```python
from build123d import *


with BuildPart() as part:
    # Эскиз2 → Повернуть1 (revolve)
    with BuildSketch(Plane.XY):
        with BuildLine():
            Line((0, 21), (0, 15))
            ThreePointArc((0, 15), (0.585786438, 13.585786438), (2, 13))
            Line((2, 13), (5, 13))
            Line((5, 13), (5, 14))
            Line((5, 14), (3, 14))
            ThreePointArc((3, 14), (1.585786438, 14.585786438), (1, 16))
            Line((1, 16), (1, 21))
            Line((1, 21), (0, 21))
        make_face()
    revolve(axis=Axis((0, 0, 0), (1, 0, 0)))


solid = part.part
```
Design review of the part built by this model. Coordinates are the model's own, in mm. A direction names the side the tool comes from. Give positions to 0.01 mm unless a question says otherwise; leave off trailing zeros. Order: outer loops, then holes, each group sorted by start corner. A loop starts at its lowest first (then second) coordinate and runs counter-clockwise, first axis right, second up. Notation, with made-up numbers: (12, 86.5) -> (25, 86.5) arc R26 ccw to (25, 104.5) -> close; hole circle Ø6 at (-16, 21.5). An arc over 180 degrees is marked (long way). Write each question's results on one line, items separated by ' | '. Start each with the question number.
Q1. Mouldability with a two-part tool opening along Y and no side actions: class faces 1 (the cylindrical face through (0.49, 20.03, 6.31)), 2 (the flat face through (1, 4.8, -15.5)), 3 (the cylindrical face through (3.521, -10.316, -7.91)) as +Y half, -Y half, draft (parallel to the pull), parting line (faces both ways), or undercut.
Q2. Machinability: for faces 4 (the cylindrical face through (3.986, 12.932, -5.362)), 5 (the flat face through (0, 9, -14)), which of the approach directions +Z, -Z, +X, -X, +Y, -Y give a long, thin tool a straight path to every point of the face, cutting with its end or side? Answer none if there is none.
Q3. Add section A-A on z = 0. Give the boundary of the cut face in (x, y), and give its area (3 significant figures).
Q4. For pin 1 (1 mm diameter, centred on x = 4.5, y = -6.5, fed in from +Z), flat-tipped, find the tip position at first contact; note if it passes through.
Q5. Add section C-C on x = 4.4. Give the boundary of the cut face in (y, z), and give its area (3 significant figures).
Q6. Wall thickness on L1, parallel to Z at x = 3.7, y = 0; L2, parallel to X at y = -9.5, z = -13; L3, parallel to Y at x = 4.35, z = -0.5: over which ranges is each line inside the solid? List them lowest first. Write a range as from..to.
Found:
1) face 1: parting line | face 2: draft | face 3: undercut
2) face 4: +X | face 5: +Z, -Z, -X, +Y, -Y
3) outline: (0, -21) -> (1, -21) -> (1, -16) arc R2 cw to (3, -14) -> (5, -14) -> (5, -13) -> (2, -13) arc R2 ccw to (0, -15) -> close; (0, 15) arc R2 ccw to (2, 13) -> (5, 13) -> (5, 14) -> (3, 14) arc R2 cw to (1, 16) -> (1, 21) -> (0, 21) -> close | area: 24.0 mm2
4) pin 1: stops at z = 12.65
5) outline: circle Ø28 at (0, 0); hole circle Ø26 at (0, 0) | area: 84.8 mm2
6) L1: z = -14..-13, 13..14 | L2: x = 0..1 | L3: y = -13.99..-12.99, 12.99..13.99
